Geometry check sheet. Reference: the model listing, model coordinates, mm. A direction names the side the tool comes from. Round coordinates to 2 decimals unless told otherwise and drop trailing zeros. Loops run counter-clockwise (first coordinate to the right, second up) from the corner with the lowest first, then second, coordinate; pieces in that order, holes last. Notation, with made-up numbers: M 46.25,33 L 93.25,33 A16 ccw 93.25,43 Z; hole C 37.5,47 d3. An arc over 180 degrees is marked long. Use one line per item in the form item = value. Start each with the question number.
1. Cross-section at C-C (x = -2.5). State how many separate pieces and enclosed holes the cut face has, then the cut area to 3 significant figures.
2. Set-up check for faces 1 (the flat face through (30, -12.5, -52)), 2 (the flat face through (54, 12.5, -34)), 3 (the flat face through (44.761, -0.175, 74.464)): record each of +Z, -Z, +X, -X, +Y, -Y from which the full face is reachable in a straight line by a thin tool's end or side.
3. Draft check along Y on faces 4 (the conical face through (9.247, 3.094, -41.642)), 5 (the conical face through (-51.889, -3.524, 31.058)), 6 (the conical face through (-48.456, 7.579, 47.762)). Enter one of: pulls with the +Y half, pulls with the -Y half, needs draft (parallel to the pull), parting line crosses it, or undercut.
4. Cross-section at B-B (y = 20). Record the boundary of the cut face in (x, z), then the cut area to 3 significant figures.
5. Go/stop test with flat-tipped pins: pin 1 (11 mm diameter, centred on x = -47.73, z = -47.73, fed in from -Y); pin 2 (6.5 mm diameter, centred on x = 47.73, z = 47.73, fed in from -Y); pin 3 (5 mm diameter, centred on x = -47.73, z = 47.73, fed in from -Y). Record where each tip stops, or that it passes through.
6. Cross-section at A-A (z = -85). Record the boundary of the cut face in (x, y).
7. Material ranges on line 1 (Z direction, x = 0, y = 1.5); line 2 (X direction, y = -15, z = 0); line 3 (Z direction, x = 51.5, y = -1), recorded low to high.
Autodesk Inventor part; units mm, degrees
ref_plane "XZ Plane" through (0, 0, 0) normal (0, 1, 0) x (-1, 0, 0)
ref_plane "XY Plane" through (0, 0, 0) normal (0, 0, 1) x (1, 0, 0)
ref_plane "Work Plane1" through (0, -0.5, 0) normal (0, 1, 0) x (1, 0, 0)
sketch "Sketch1" plane through (0, 0, 0) normal (0, 1, 0) x (-1, 0, 0)
  line L0 (64.6952, -47.0588) -> (24.2607, -102.6471)
  arc A0 (-24.2607, -102.6471) -> (24.2607, -102.6471) centre (0, -85) ccw
  line L1 (-24.2607, -102.6471) -> (-64.6952, -47.0588)
  arc A1 (-64.6952, 47.0588) -> (-64.6952, -47.0588) centre (0, 0) ccw
  line L2 (-64.6952, 47.0588) -> (-24.2607, 102.6471)
  arc A2 (24.2607, 102.6471) -> (-24.2607, 102.6471) centre (0, 85) ccw
  line L3 (24.2607, 102.6471) -> (64.6952, 47.0588)
  arc A3 (64.6952, -47.0588) -> (64.6952, 47.0588) centre (0, 0) ccw
  dimension "d0" = 170
  dimension "d1" = 160
  dimension "d3" = 30
extrude "Extrusion1" add sketch "Sketch1" along normal mid plane 25
sketch "Sketch2" plane through (0, 12.5, 0) normal (0, 1, 0) x (1, 0, 0)
  arc A0 (24.2607, 102.6471) -> (-24.2607, 102.6471) centre (0, 85) ccw
  arc A1 (-24.2607, -102.6471) -> (24.2607, -102.6471) centre (0, -85) ccw
hole "Hole1" at (0, 12.5, -85) at (0, 12.5, 85) direction (0, -1, 0) diameter 26 end through all
sketch "Sketch3" plane through (0, 0, 0) normal (0, 0, 1) x (1, 0, 0)
  line L0 (0, 37.5) -> (0, -20.5)
  line L1 (0, 37.5) -> (-61, 37.5)
  line L2 (-61, 37.5) -> (-61, -12.5)
  line L3 (-64.6952, -12.5) -> (-24.2607, -12.5)
  line L4 (-61, -12.5) -> (-57.5, -12.5)
  line L5 (-57.5, -12.5) -> (-57.5, -20.5)
  line L6 (-57.5, -20.5) -> (0, -20.5)
  line L7 (-24.2607, 12.5) -> (-64.6952, 12.5)
  point P0 (0, 0)
  dimension "d13" = 58
  dimension "d14" = 122
  dimension "d15" = 115
  dimension "d16" = 25
revolve "Revolution1" add sketch "Sketch3" angle 360 about axis through (0, 37.5, 0) along (0, -1, 0)
sketch "Sketch4" plane through (0, 0, 0) normal (0, 0, 1) x (1, 0, 0)
  line L0 (0, -20.5) -> (0, 37.5)
  line L1 (-61, 37.5) -> (61, 37.5)
  line L2 (0, 37.5) -> (-51, 37.5)
  line L3 (-51, 37.5) -> (-51, 4.5)
  line L4 (-51, 4.5) -> (-45, 4.5)
  line L5 (-42.5, 3) -> (-42.5, -0.5)
  line L6 (-42.5, -0.5) -> (-45, -0.5)
  line L7 (-45, -0.5) -> (-45, -20.5)
  line L8 (-57.5, -20.5) -> (57.5, -20.5)
  line L9 (-45, -20.5) -> (0, -20.5)
  line L10 (-45, 4.5) -> (-42.5, 3)
  point P0 (0, 0)
  dimension "d18" = 102
  dimension "d19" = 90
  dimension "d20" = 85
  dimension "d21" = 33
  dimension "d22" = 20
  dimension "d23" = 1.5
  dimension "d24" = 90
revolve "Revolution2" cut sketch "Sketch4" angle 360 about axis through (0, -20.5, 0) along (0, 1, 0)
hole "Hole2" at (-69.282, -0.5, 40) direction (0.8660254, 0, -0.5) diameter 6 end up to surface
hole "Hole3" at (-69.282, -0.5, 40) direction (0.8660254, 0, -0.5) diameter 11.445 depth 18 tip angle 118
thread "Thread1"
sketch "Sketch5" plane through (0, -12.5, 0) normal (0, -1, 0) x (1, 0, 0)
  arc A0 (64.6952, -47.0588) -> (64.6952, 47.0588) centre (0, 0) ccw
  line L0 (0, 0) -> (47.7297, 47.7297) construction
  line L1 (0, 0) -> (67.5, 0) construction
  dimension "d48" = 67.5
  dimension "d49" = 45
hole "Hole4" at (47.7297, -12.5, 47.7297) direction (0, 1, 0) diameter 8.376 depth 18 tip angle 118
pattern_circular "Circular Pattern1" count 4 over 360 about axis through (0, -16.5, 0) along (0, -1, 0) of "Hole4"
fillet "Fillet1" radius 2 2 edges at (61, 12.5, 0) (57.5, -12.5, 0)
chamfer "Chamfer1" distance 1 angle 45 6 edges at (57.5, -20.5, 0) (45, -20.5, 0) (61, 37.5, 0) (51, 37.5, 0) (-41.4147, -0.5, 9.5432) (40.6378, -0.5, -12.4427)
ref_plane "Work Plane1" through (0, -0.5, 0) normal (0, 1, 0) x (1, 0, 0)
ref_plane "Work Plane2" through (0, 0, 0) normal (-0.5, 0, -0.8660254) x (0, 1, 0)
properties part number "Part037. Main arbor flange" material "Steel, Carbon"
Reported:
q1.separate_pieces = 4
q1.enclosed_holes = 0
q1.area = 2,850 mm²
q2.face_1 = -Y
q2.face_2 = +Y
q2.face_3 = +Z, +X, +Y, -Y
q3.face_4 = pulls with the +Y half
q3.face_5 = undercut
q3.face_6 = pulls with the -Y half
q4.outline = C 0,0 d122; hole C 0,0 d102
q4.area = 3,520 mm²
q5.pin_1 = -12.5
q5.pin_2 = 6.06
q5.pin_3 = 6.51
q6.outline = M -37.1,-12.5 L -13,-12.5 L -13,12.5 L -37.1,12.5 Z; M 13,-12.5 L 37.1,-12.5 L 37.1,12.5 L 13,12.5 Z
q7.line_1 = -115 to -98, -72 to -42.5, 42.5 to 72, 98 to 115
q7.line_2 = -57.5 to -45, 45 to 57.5
q7.line_3 = -65.2 to -49.55, -45.91 to 45.91, 49.55 to 65.2
